from build123d import *

# Parameters (mm, degrees)
ESBO_O1_R                = 3
RESSALTO_EXTRUS_O1_DEPTH = 77
CORTE_EXTRUS_O1_START    = -4
ESBO_O2_R                = 3
ESBO_O2_R_2              = 2
CORTE_EXTRUS_O1_DEPTH    = 4
ESBO_O3_R                = 3
ESBO_O3_R_2              = 2
CORTE_EXTRUS_O2_DEPTH    = 20
ESBO_O4_R                = 2.5
ESBO_O4_R_2              = 1.5
CORTE_EXTRUS_O3_DEPTH    = 16


with BuildPart() as part:
    # Esboço1 → Ressalto-extrusão1 (new body)
    with BuildSketch(Plane.XY):
        Circle(ESBO_O1_R)
    extrude(amount=RESSALTO_EXTRUS_O1_DEPTH)

    # Esboço2 → Corte-extrusão1 (cut)
    with BuildSketch(Plane.XY.offset(77).offset(CORTE_EXTRUS_O1_START)):
        Circle(ESBO_O2_R)
        Circle(ESBO_O2_R_2, mode=Mode.SUBTRACT)
    extrude(amount=CORTE_EXTRUS_O1_DEPTH, mode=Mode.SUBTRACT)

    # Esboço3 → Corte-extrusão2 (cut)
    with BuildSketch(Plane(origin=(0, 0, 0), x_dir=(-1, 0, 0), z_dir=(0, 0, -1))):
        with Locations(Location((0, 0, 0), (0, 0, 180))):
            Circle(ESBO_O3_R)
        with Locations(Location((0, 0, 0), (0, 0, 180))):
            Circle(ESBO_O3_R_2, mode=Mode.SUBTRACT)
    extrude(amount=-CORTE_EXTRUS_O2_DEPTH, mode=Mode.SUBTRACT)

    # Esboço4 → Corte-extrusão3 (cut)
    with BuildSketch(Plane(origin=(0, 0, 0), x_dir=(-1, 0, 0), z_dir=(0, 0, -1))):
        Circle(ESBO_O4_R)
        Circle(ESBO_O4_R_2, mode=Mode.SUBTRACT)
    extrude(amount=-CORTE_EXTRUS_O3_DEPTH, mode=Mode.SUBTRACT)


solid = part.part
Read the model definition and answer for the solid it produces. Units are mm, in the model's axes. A direction names the side the tool comes from. Give positions to 0.01 mm unless a question says otherwise; leave off trailing zeros. Write each loop counter-clockwise with the first axis right and the second up, starting at its lowest first coordinate (ties: lowest second). Pieces come first, ordered by that corner, then holes. Notation, with made-up numbers: (-34.5, -16) - (-15.5, -16) arc R29 cw to (-15.5, 5) - close; hole circle Ø9 at (68.25, 63). An arc over 180 degrees is marked (long way). Answer in a Markdown table with one row per item. Add a question column.
Item 1: Section D-D, the plane z = 7 is taken. Write down the section's boundary in (x, y), and give its area (3 significant figures).
Item 2: Section C-C, the plane z = 22 is taken. Write down the section's boundary in (x, y), and give its area (3 significant figures).
Item 3: Find the intervals of material crossed by L1, parallel to Z at x = -2.6, y = 0.65; L2, parallel to X at y = -0.15, z = 42.5; L3, parallel to Y at x = -0.3, z = 58.5, in increasing order.
Item 4: Section A-A, the plane y = 0 is taken. Write down the section's boundary in (x, z), and give its area (3 significant figures).
Item 5: A tool of negligible diameter and unlimited length cuts with its end or side. For faces 1 (the face through (0, 0, 0)), 2 (the face through (1, -2, 73)), 3 (the face through (0, 2, 18)), from which of +Z, -Z, +X, -X, +Y, -Y can it reach the whole face along a straight path? Write none if from no direction.
Item 6: Flat-ended cylindrical pins translate along their axes: P1, Ø1.8, axis at x = 0.5, y = -1, coming from the -Z side; P2, Ø2, axis at x = 0, z = 11, coming from the -Y side; P3, Ø1, axis at x = -2, z = 42, coming from the +Y side; P4, Ø2, axis at y = 2, z = 53, coming from the +X side. Find the tip coordinate at first contact, or state that the pin passes through.
Recorded:
| question | item | result |
|---|---|---|
| 1 | outline | circle Ø3 at (0, 0) |
| 1 | area | 7.07 mm2 |
| 2 | outline | circle Ø6 at (0, 0) |
| 2 | area | 28.3 mm2 |
| 3 | L1 | z = 20 to 73 |
| 3 | L2 | x = -3 to 3 |
| 3 | L3 | y = -2.98 to 2.98 |
| 4 | outline | (-3, 20) - (-2, 20) - (-2, 16) - (-1.5, 16) - (-1.5, 0) - (1.5, 0) - (1.5, 16) - (2, 16) - (2, 20) - (3, 20) - (3, 73) - (2, 73) - (2, 77) - (-2, 77) - (-2, 73) - (-3, 73) - close |
| 4 | area | 398 mm2 |
| 5 | face 1 | -Z, +X, -X, +Y, -Y |
| 5 | face 2 | +Z |
| 5 | face 3 | -Z |
| 6 | P1 | stops at z = 0 |
| 6 | P2 | stops at y = -1.5 |
| 6 | P3 | stops at y = 2.6 |
| 6 | P4 | stops at x = 2.83 |
